Geometry: final body of the model. Coordinates: model frame, mm. A direction names the side the tool comes from. Give positions to 0.01 mm unless a question says otherwise; leave off trailing zeros. Loops run counter-clockwise (first coordinate to the right, second up) from the corner with the lowest first, then second, coordinate; pieces in that order, holes last.
1. Section A-A, the plane x = 0. State how many separate pieces and enclosed holes the cut face has, then the cut area to 3 significant figures.
2. First-contact query: P1, Ø8, axis at x = 22.5, y = 33, coming from the +Z side; P2, Ø4, axis at x = -10.5, z = 118, coming from the +Y side; P3, Ø1.5, axis at x = 23, z = 140.5, coming from the +Y side; P4, Ø4, axis at x = 24.5, y = 33.5, coming from the -Z side. Flat tips, straight axial feed; report the tip coordinate or a pass-through.
3. Material intervals for line 1 along Y through (x, z) = (0, 162.5); line 2 along Z through (x, y) = (0, 31) (1 decimal); line 3 along Y through (x, z) = (0, 53), sorted ascending.
4. Section C-C, the plane y = -22.5. Output: boundary loops of the cut face in (x, z) (3 decimals), then the cut area to 3 significant figures.
5. Access query for faces 1 (the face through (28, -12, 0)), 2 (the face through (24.636, 29.9, 97.527)), 3 (the face through (-5.782, -26.036, 88.179)), 4 (the face through (30.133, 1.326, 12.522)), 5 (the face through (0, -27, 149.225)). Directions: +Z, -Z, +X, -X, +Y, -Y. A direction counts if a zero-diameter tool reaches every point of the face in a straight line with its end or side. Return the directions, or none.
6. Section B-B, the plane z = 32.5. Output: boundary loops of the cut face in (x, y).
7. Draft query along X for faces 6 (the face through (-4.13, -31.48, 86.09)), 7 (the face through (28, -12, 174.625)), 8 (the face through (0, -27, 25.4)). Return one class per face: +X half, -X half, draft (parallel to the pull), parting line (faces both ways), or undercut.
Autodesk Inventor part; units mm, degrees
ref_plane "Work Plane5" through (0, 31.75, 174.625) normal (0, 1, 0) x (-1, 0, 0)
ref_plane "Work Plane6" through (31.496, 0, 0) normal (1, 0, 0) x (0, 1, 0)
ref_plane "XZ Plane" through (0, 0, 0) normal (0, 1, 0) x (-1, 0, 0)
sketch "Sketch1" plane through (0, 0, 0) normal (0, 0, 1) x (1, 0, 0)
  circle A0 centre (0, 0) radius 31.75
  dimension "d0" = 63.5
extrude "mainBody" add sketch "Sketch1" along normal blind 174.625
sketch "Sketch10" plane through (0, 0, 174.625) normal (0, 0, 1) x (1, 0, 0)
  circle A0 centre (0, 0) radius 30.1625
  circle A1 centre (0, 0) radius 31.75
  point P0 (0, 31.75)
ref_plane "Work Plane5" through (0, 31.75, 174.625) normal (0, 1, 0) x (-1, 0, 0)
sketch "Sketch11" plane through (0, 31.75, 174.625) normal (0, 1, 0) x (-1, 0, 0)
  circle A0 centre (0, -87.3125) radius 31.75
  line L0 (31.75, 0) -> (-31.75, 0)
  point P0 (0, -174.625)
  dimension "d29" = 87.3125
  dimension "d30" = 63.5
extrude "TBody" add sketch "Sketch11" along normal blind 38.1 and the other way blind 31.75
sketch "Sketch12" plane through (0, 69.85, 87.3125) normal (0, 1, 0) x (1, 0, 0)
  circle A0 centre (0, 0) radius 31.75
  circle A1 centre (0, 0) radius 30.1625
  point P0 (0, 87.3125)
  dimension "d35" = 60.325
extrude "TSocket" cut sketch "Sketch12" against normal blind 25.4 contours A1
sketch "Sketch13" plane through (0, 44.45, 87.3125) normal (0, 1, 0) x (1, 0, 0)
  circle A0 centre (0, 0) radius 30.1625
  circle A1 centre (0, 0) radius 26.67
  point P0 (0, 87.3125)
  dimension "d39" = 53.34
extrude "TTube" cut sketch "Sketch13" against normal blind 38.1 contours A1
sketch "Sketch14" plane through (0, 0, 174.625) normal (0, 0, 1) x (1, 0, 0)
  circle A0 centre (0, 0) radius 31.75
  circle A1 centre (0, 0) radius 26.67
  dimension "d43" = 53.34
extrude "mainTube" cut sketch "Sketch14" against normal blind 177.8 contours A1
sketch "Sketch15" plane through (0, 0, 174.625) normal (0, 0, 1) x (1, 0, 0)
  circle A0 centre (0, 0) radius 26.67
  circle A1 centre (0, 0) radius 31.75
  circle A2 centre (0, 0) radius 30.1625
  dimension "d47" = 60.325
extrude "mainSocket1" cut sketch "Sketch15" against normal blind 25.4 contours A2
sketch "Sketch16" plane through (0, 0, 0) normal (0, 0, -1) x (-1, 0, 0)
  circle A0 centre (0, 0) radius 26.67
  circle A1 centre (0, 0) radius 31.75
  circle A2 centre (0, 0) radius 30.1625
  dimension "d51" = 60.325
extrude "mainSocket2" cut sketch "Sketch16" against normal blind 25.4 contours A2
sketch "Sketch24" plane through (0, 69.85, 87.3125) normal (0, 1, 0) x (1, 0, 0)
  circle A0 centre (0, 0) radius 30.1625
  line L0 (-30.1625, 0) -> (30.1625, 0) construction
  line L1 (0, 30.1625) -> (0, -30.1625) construction
  line L2 (-30.9225, -1.27) -> (-28.3825, -1.27)
  line L3 (-28.3825, -1.27) -> (-28.3825, 1.27)
  line L4 (-28.3825, 1.27) -> (-30.9225, 1.27)
  line L5 (-30.9225, 1.27) -> (-30.9225, -1.27)
  line L6 (-30.9225, 0) -> (-28.3825, 0) construction
  line L7 (30.9225, -1.27) -> (28.3825, -1.27)
  line L8 (28.3825, -1.27) -> (28.3825, 1.27)
  line L9 (28.3825, 1.27) -> (30.9225, 1.27)
  line L10 (30.9225, 1.27) -> (30.9225, -1.27)
  line L11 (30.9225, 0) -> (28.3825, 0) construction
  point P0 (0, 87.3125)
  dimension "d72" = 2.54
  dimension "d75" = 2.54
extrude "Extrusion20" cut sketch "Sketch24" against normal blind 25.4 contours A0 L7 L8 L9 | A0 L9 L10 L7 | L4 L3 L2 A0 | A0 L2 L5 L4
ref_plane "Work Plane6" through (31.496, 0, 0) normal (1, 0, 0) x (0, 1, 0)
sketch "Sketch27" plane through (31.496, 0, 0) normal (1, 0, 0) x (0, 1, 0)
  line L0 (-1.5232, -1.2223) -> (1.5232, -1.2223)
  line L1 (1.5232, -1.2223) -> (1.5232, 8.0295)
  line L2 (1.5232, 8.0295) -> (-1.5232, 8.0295)
  line L3 (-1.5232, 8.0295) -> (-1.5232, -1.2223)
  point P0 (0, 0)
extrude "Extrusion22" cut sketch "Sketch27" along normal blind 25.4
properties part number "0pvc_T_2in" material "PVC-Piping"
Answers below:
1. separate pieces: 3
1. enclosed holes: 0
1. area: 1,360 mm2
2. P1: stops at z = 113.12
2. P2: stops at y = 69.85
2. P3: stops at y = 22.65
2. P4: stops at z = 64.91
3. line 1: y = -31.75 to -30.16, 30.16 to 31.75
3. line 2: z = 0 to 60.6, 114 to 174.6
3. line 3: y = -31.75 to -26.67, 26.67 to 31.75
4. outline: (-22.401, 0) - (-20.088, 0) - (-20.088, 25.4) - (-14.319, 25.4) - (-14.319, 149.225) - (-20.088, 149.225) - (-20.088, 174.625) - (-22.401, 174.625) - close; (14.319, 25.4) - (20.088, 25.4) - (20.088, 0) - (22.401, 0) - (22.401, 174.625) - (20.088, 174.625) - (20.088, 149.225) - (14.319, 149.225) - close
4. area: 2,240 mm2
5. face 1: -Z, +X, -X, +Y, -Y
5. face 2: +Y
5. face 3: +Z, -Z
5. face 4: -Z
5. face 5: +Z
6. outline: circle Ø63.5 at (0, 0); hole circle Ø53.34 at (0, 0)
7. face 6: parting line
7. face 7: draft
7. face 8: undercut
